```python
from build123d import *

# Parameters (mm, degrees)
F0_W     = 19
F0_H     = 19
F1_DEPTH = 9.5
F3_START = -2
F2_W     = 15
F2_H     = 15
F3_DEPTH = 15
F5_R     = 1
F4_R     = 1.5
F6_DEPTH = 2


with BuildPart() as f1:
    # F0 (on Top) → F1 (new body, symmetric)
    with BuildSketch(Plane.XY):
        Rectangle(F0_W, F0_H)
    extrude(amount=F1_DEPTH, both=True)

    # F2 (on face) → F3 (cut)
    with BuildSketch(Plane(origin=(-9.5, 0, 0), x_dir=(0, -1, 0), z_dir=(-1, 0, 0)).offset(F3_START)):
        Rectangle(F2_W, F2_H)
    extrude(amount=-F3_DEPTH, mode=Mode.SUBTRACT)

    # F5
    f5_edges = [f1.edges().sort_by_distance(p)[0] for p in [
        (-9.5, 0, 9.5),
        (0, -9.5, 9.5),
        (9.5, 0, 9.5),
        (0, 9.5, 9.5),
        (-9.5, 9.5, 0),
        (9.5, 9.5, 0),
        (0, 9.5, -9.5),
        (9.5, -9.5, 0),
        (0, -9.5, -9.5),
        (9.5, 0, -9.5),
        (-9.5, -9.5, 0),
        (-9.5, 0, -9.5),
    ]]
    fillet(f5_edges, radius=F5_R)

    # F4 (on face) → F6 (cut)
    with BuildSketch(Plane(origin=(-9.5, 0, 0), x_dir=(0, -1, 0), z_dir=(-1, 0, 0))):
        Circle(F4_R)
    extrude(amount=-F6_DEPTH, mode=Mode.SUBTRACT)


solid = f1.part
```
Here's how the part is built. I have some questions about the finished solid (model axes, mm). A direction names the side the tool comes from. Round coordinates to 2 decimals unless told otherwise and drop trailing zeros. Write each loop counter-clockwise with the first axis right and the second up, starting at its lowest first coordinate (ties: lowest second). Pieces come first, ordered by that corner, then holes.
Q1. Will this pin go through, and if not, where does the flat tip stop? P1, Ø1.8, axis at y = 0, z = 0, coming from the -X side.
Q2. If we mould it in two halves opening along Y, with no side actions, what happens to faces 3 (the flat face through (0, -9.5, 0)), 4 (the cylindrical face through (0.119, 9.199, -9.215)), 5 (the flat face through (7.5, 0, 0))? For each: +Y half, -Y half, draft (parallel to the pull), parting line (faces both ways), or undercut.
Q3. Which directions (+Z, -Z, +X, -X, +Y, -Y) give clear straight access to the entire face, cutting with the end or side of a thin tool? Please do faces 1 (the flat face through (0, 7.5, 0)), 2 (the cylindrical face through (0.119, 9.215, 9.199)).
Q4. If we section it at C-C on z = 0: Write out the boundary of the cut face in (x, y).
Q5. If we section it at A-A on z = -6.5: Write out the boundary of the cut face in (x, y), plus the area to 3 significant figures.
Q6. Please list where these lines run through material, in increasing order: probe 1 along Z at (x, y) = (-1, -7); probe 2 along Z at (x, y) = (-8.1, 0).
Answer below:
1. P1: stops at x = 7.5
2. face 3: -Y half
2. face 4: +Y half
2. face 5: undercut
3. face 1: none
3. face 2: +Z, +X, -X, +Y
4. outline: (-9.5, -8.5) arc R1 ccw to (-8.5, -9.5) - (8.5, -9.5) arc R1 ccw to (9.5, -8.5) - (9.5, 8.5) arc R1 ccw to (8.5, 9.5) - (-8.5, 9.5) arc R1 ccw to (-9.5, 8.5) - (-9.5, 1.5) - (-7.5, 1.5) - (-7.5, 7.5) - (7.5, 7.5) - (7.5, -7.5) - (-7.5, -7.5) - (-7.5, -1.5) - (-9.5, -1.5) - close
5. outline: (-9.5, -8.5) arc R1 ccw to (-8.5, -9.5) - (8.5, -9.5) arc R1 ccw to (9.5, -8.5) - (9.5, 8.5) arc R1 ccw to (8.5, 9.5) - (-8.5, 9.5) arc R1 ccw to (-9.5, 8.5) - close; hole (-7.5, -7.5) - (7.5, -7.5) - (7.5, 7.5) - (-7.5, 7.5) - close
5. area: 135 mm2
6. probe 1: z = -9.5 to -7.5, 7.5 to 9.5
6. probe 2: z = -9.5 to -1.5, 1.5 to 9.5
